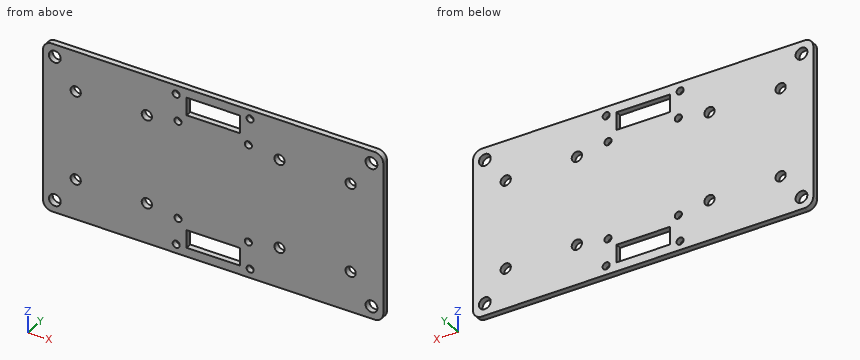
from build123d import *

# Parameters (mm, degrees)
ESBO_O1_W                = 115.09677689
ESBO_O1_H                = 57
RESSALTO_EXTRUS_O1_DEPTH = 2
ESBO_O2_R                = 1.73
CORTE_EXTRUS_O1_DEPTH    = 65.699822354
ESBO_O3_W                = 18
ESBO_O3_H                = 6
CORTE_EXTRUS_O2_DEPTH    = 65.699822354
ESBO_O5_R                = 2
CORTE_EXTRUS_O3_DEPTH    = 65.699822354
FILETE1_R                = 3
ESBO_O8_R                = 1.2
CORTE_EXTRUS_O4_DEPTH    = 65.699822354


with BuildPart() as part:
    # Esboço1 → Ressalto-extrusão1 (new body)
    with BuildSketch(Plane(origin=(0, 0, 0), x_dir=(1, 0, 0), z_dir=(0, 1, 0))):
        with Locations((0, 1)):
            Rectangle(ESBO_O1_W, ESBO_O1_H)
    extrude(amount=RESSALTO_EXTRUS_O1_DEPTH)

    # Esboço2 → Corte-extrusão1 (cut, through all)
    with BuildSketch(Plane(origin=(0, 2, 0), x_dir=(1, 0, 0), z_dir=(0, 1, 0))):
        with Locations(Location((-46.488388445, 15.945, 0), (0, 0, 270))):
            Circle(ESBO_O2_R)
        with Locations(Location((-22.428388445, 15.945, 0), (0, 0, 270))):
            Circle(ESBO_O2_R)
        with Locations(Location((-22.428388445, -13.945, 0), (0, 0, 270))):
            Circle(ESBO_O2_R)
        with Locations(Location((22.428388445, -13.945, 0), (0, 0, 90))):
            Circle(ESBO_O2_R)
        with Locations(Location((22.428388445, 15.945, 0), (0, 0, 90))):
            Circle(ESBO_O2_R)
        with Locations(Location((46.488388445, 15.945, 0), (0, 0, 90))):
            Circle(ESBO_O2_R)
        with Locations(Location((-46.488388445, -13.945, 0), (0, 0, 270))):
            Circle(ESBO_O2_R)
        with Locations(Location((46.488388445, -13.945, 0), (0, 0, 90))):
            Circle(ESBO_O2_R)
    extrude(amount=-CORTE_EXTRUS_O1_DEPTH, mode=Mode.SUBTRACT)

    # Esboço3 → Corte-extrusão2 (cut, through all)
    with BuildSketch(Plane.XZ):
        with Locations((0, 21.5)):
            Rectangle(ESBO_O3_W, ESBO_O3_H)
        with Locations((0, -23.5)):
            Rectangle(ESBO_O3_W, ESBO_O3_H)
    extrude(amount=-CORTE_EXTRUS_O2_DEPTH, mode=Mode.SUBTRACT)

    # Esboço5 → Corte-extrusão3 (cut, through all)
    with BuildSketch(Plane(origin=(0, 2, 0), x_dir=(1, 0, 0), z_dir=(0, 1, 0))):
        with Locations(Location((53.548388445, 25.3375, 0), (0, 0, 270))):
            Circle(ESBO_O5_R)
        with Locations(Location((53.548388445, -23.3375, 0), (0, 0, 90))):
            Circle(ESBO_O5_R)
        with Locations(Location((-53.548388445, -23.3375, 0), (0, 0, 270))):
            Circle(ESBO_O5_R)
        with Locations(Location((-53.548388445, 25.3375, 0), (0, 0, 90))):
            Circle(ESBO_O5_R)
    extrude(amount=-CORTE_EXTRUS_O3_DEPTH, mode=Mode.SUBTRACT)

    # Filete1
    filete1_edges = [part.edges().sort_by_distance(p)[0] for p in [
        (-57.548388445, 1, -29.5),
        (57.548388445, 1, -29.5),
        (57.548388445, 1, 27.5),
        (-57.548388445, 1, 27.5),
    ]]
    fillet(filete1_edges, radius=FILETE1_R)

    # Esboço8 → Corte-extrusão4 (cut, through all)
    with BuildSketch(Plane(origin=(0, 2, 0), x_dir=(1, 0, 0), z_dir=(0, 1, 0))):
        with Locations(Location((-12.498388445, 26.5, 0), (0, 0, 270))):
            Circle(ESBO_O8_R)
        with Locations(Location((12.498388445, 26.5, 0), (0, 0, 90))):
            Circle(ESBO_O8_R)
        with Locations(Location((12.498388445, -24.5, 0), (0, 0, 270))):
            Circle(ESBO_O8_R)
        with Locations(Location((-12.498388445, -24.5, 0), (0, 0, 90))):
            Circle(ESBO_O8_R)
        with Locations(Location((-11.898388445, 17.5, 0), (0, 0, 270))):
            Circle(ESBO_O8_R)
        with Locations(Location((11.898388445, 17.5, 0), (0, 0, 90))):
            Circle(ESBO_O8_R)
        with Locations(Location((11.898388445, -15.5, 0), (0, 0, 270))):
            Circle(ESBO_O8_R)
        with Locations(Location((-11.898388445, -15.5, 0), (0, 0, 90))):
            Circle(ESBO_O8_R)
    extrude(amount=-CORTE_EXTRUS_O4_DEPTH, mode=Mode.SUBTRACT)


solid = part.part
Can you work these out from the model? Positions are in its coordinate system, mm. Give positions to 0.01 mm unless a question says otherwise; leave off trailing zeros. Order: outer loops, then holes, each group sorted by start corner. A loop starts at its lowest first (then second) coordinate and runs counter-clockwise, first axis right, second up. Notation, with made-up numbers: M 29,49 L 79,49 A7 cw 79,61 Z; hole C 31.25,42 d11. An arc over 180 degrees is marked long. Use a Markdown table: item, result. Add a question column.
Item 1: If I drill on L1, parallel to Z at x = 7, y = 0.5; L2, parallel to Z at x = 45.5, y = 0.7; L3, parallel to X at y = 1.7, z = 12.5, over which ranges is the centre line in solid material (lowest first)? Write a range as [from, to].
Item 2: Will these pins go through, and if not, where does the flat tip stop? pin 1 (10 mm diameter, centred on x = -3, z = -2, fed in from -Y); pin 2 (3 mm diameter, centred on x = -46.49, z = 13.94, fed in from -Y).
Item 3: Suppose I cut it at A-A (x = 5.5). List the corners of the cut face in (y, z) for me, then the cut area to 3 significant figures.
Item 4: Suppose I cut it at B-B (y = 1.2). Count the separate pieces of the cut face and the enclosed holes in it, then the cut area to 3 significant figures.
Answer sheet:
| question | item | result |
|---|---|---|
| 1 | L1 | z = [-29.5, -26.5], [-20.5, 18.5], [24.5, 27.5] |
| 1 | L2 | z = [-29.5, -17.36], [-14.53, 12.53], [15.36, 27.5] |
| 1 | L3 | x = [-57.55, -47.44], [-45.54, -23.38], [-21.48, 21.48], [23.38, 45.54], [47.44, 57.55] |
| 2 | pin 1 | stops at y = 0 |
| 2 | pin 2 | passes through |
| 3 | outline | M 0,-29.5 L 2,-29.5 L 2,-26.5 L 0,-26.5 Z; M 0,-20.5 L 2,-20.5 L 2,18.5 L 0,18.5 Z; M 0,24.5 L 2,24.5 L 2,27.5 L 0,27.5 Z |
| 3 | area | 90.0 mm² |
| 4 | separate pieces | 1 |
| 4 | enclosed holes | 22 |
| 4 | area | 6,180 mm² |
